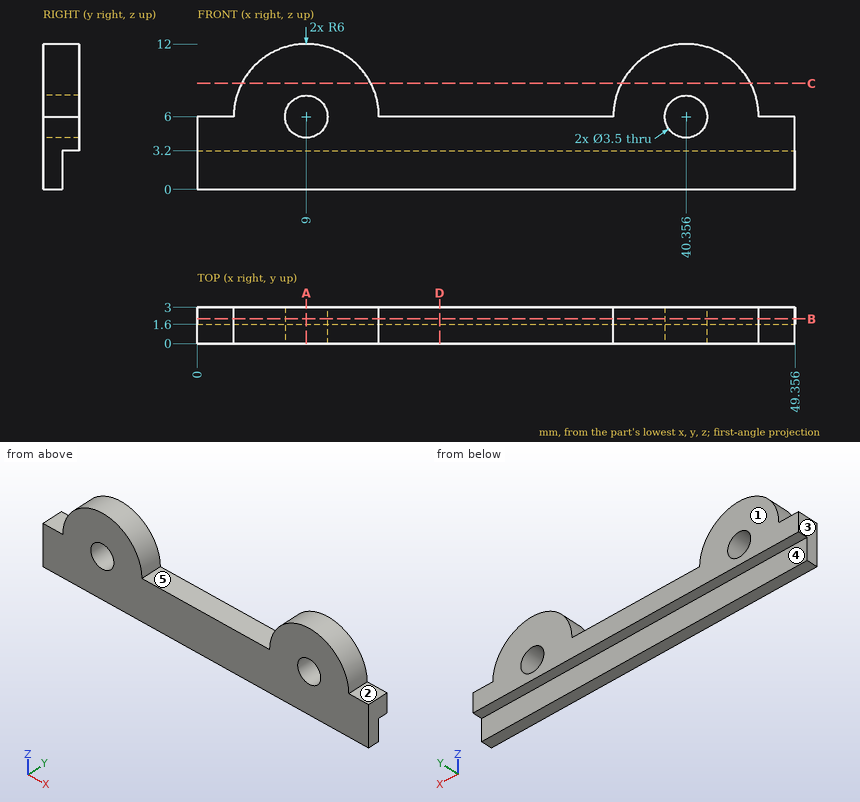
Job drawing, mm, ordinate dimensions from the low corner. One solid piece. A direction names the side the tool comes from. Round coordinates to 2 decimals unless told otherwise and drop trailing zeros. Loops run counter-clockwise (first coordinate to the right, second up) from the corner with the lowest first, then second, coordinate; pieces in that order, holes last. Notation, with made-up numbers: M 57.5,34.25 L 104.5,34.25 A21 ccw 104.5,43.25 Z; hole C 46,-27 d4. An arc over 180 degrees is marked long. One line per question, with ' | ' between items. Start each with the question number.
Item 1: Wall check: line 1 (X direction, y = 1.3, z = 5.5); line 2 (X direction, y = 1, z = 7) (1 decimal); line 3 (X direction, y = 1.65, z = 4.75) (1 decimal). Give the ranges that are in metal, low to high.
Item 2: Cut at A-A, the plane x = 9. Write the cut outline in (y, z).
Item 3: Pin check, flat tips, straight feed: pin 1 Ø1.5 at (x, y) = (48, 1) entering from +Z; pin 2 Ø0.7 at (x, y) = (22.5, 2) entering from -Z; pin 3 Ø2.5 at (x, z) = (24.5, 1) entering from +Y. Stop position of each tip, or through.
Item 4: Which spindle directions (+Z, -Z, +X, -X, +Y, -Y) get a long thin tool onto all of the face, cutting with end or side? Do the marked faces 1 and 2. Say none if no direction does.
Item 5: Cut at D-D, the plane x = 20. Write the cut outline in (y, z).
Item 6: Two-plate mould, pull along X, no slides. Class the marked faces 3, 4 and 5: pulls with the +X half, pulls with the -X half, needs draft (parallel to the pull), parting line crosses it, or undercut.
Item 7: Cut at B-B, the plane y = 2.05. Write the cut outline in (x, z).
Item 8: Cut at C-C, the plane z = 8.75. Write the cut outline in (x, y).
Responses:
1) line 1: x = 0 to 7.32, 10.68 to 38.68, 42.03 to 49.36 | line 2: x = 3.1 to 7.6, 10.4 to 14.9, 34.4 to 38.9, 41.8 to 46.3 | line 3: x = 0 to 7.8, 10.2 to 39.1, 41.6 to 49.4
2) outline: M 0,0 L 1.6,0 L 1.6,3.2 L 3,3.2 L 3,4.25 L 0,4.25 Z; M 0,7.75 L 3,7.75 L 3,12 L 0,12 Z
3) pin 1: stops at z = 6 | pin 2: stops at z = 3.2 | pin 3: stops at y = 1.6
4) face 1: +Z, -Z, +X, -X, +Y | face 2: +Z, +X, +Y, -Y
5) outline: M 0,0 L 1.6,0 L 1.6,3.2 L 3,3.2 L 3,6 L 0,6 Z
6) face 3: pulls with the -X half | face 4: needs draft | face 5: undercut
7) outline: M 0,3.2 L 49.36,3.2 L 49.36,6 L 46.36,6 A6 ccw 34.36,6 L 15,6 A6 ccw 3,6 L 0,6 Z; hole C 9,6 d3.5; hole C 40.36,6 d3.5
8) outline: M 3.67,0 L 14.33,0 L 14.33,3 L 3.67,3 Z; M 35.02,0 L 45.69,0 L 45.69,3 L 35.02,3 Z
